Geometry check sheet. Reference: the model listing, model coordinates, mm. A direction names the side the tool comes from. Coordinates: 2 decimals unless noted, no trailing zeros. Write each loop counter-clockwise with the first axis right and the second up, starting at its lowest first coordinate (ties: lowest second). Pieces come first, ordered by that corner, then holes. Notation, with made-up numbers: (5.5, 60.25) -> (48.5, 60.25) arc R16 cw to (48.5, 64.25) -> close; hole circle Ø10 at (23.25, 41). An arc over 180 degrees is marked (long way). Answer in a Markdown table with one row per item. Add a question column.
Q1. Section check A-A, the plane z = -93. Record the boundary of the cut face in (x, y), and give its area (3 significant figures).
Q2. Tool access check on faces 1 (the face through (0, 12, -108)), 2 (the face through (-51.302, 11.832, -102.915)), 3 (the face through (72.5, 12, -38)). Record the directions out of +Z, -Z, +X, -X, +Y, -Y that give a thin tool (end or side, any length) a straight path to the whole face; none if there is none.
Q3. Section check C-C, the plane y = 13. Record the boundary of the cut face in (x, z), and give its area (3 significant figures).
Q4. Release check for a two-part mould opening along X. For faces 4 (the face through (48.698, 11.832, -102.915)), 5 (the face through (1, 0, -62)), 6 (the face through (-72.5, 12, -37)) record: pulls with the +X half, pulls with the -X half, needs draft (parallel to the pull), parting line crosses it, or undercut.
Q5. Thickness scan on line 1 (X direction, y = 16.75, z = -93); line 2 (Z direction, x = 50, y = 9.5); line 3 (X direction, y = 11, z = -99.5). Record the ranges inside material, lowest first.
Q6. Section check D-D, the plane z = -111. Record the boundary of the cut face in (x, y).
Q7. Gauge pin test, flat ends, axial feed: P1, Ø12, axis at x = 59.5, y = 6.5, coming from the -Z side; P2, Ø7, axis at y = 14, z = -23, coming from the +X side; P3, Ø10, axis at y = 17.5, z = -104, coming from the -X side; P4, Ø3, axis at x = 0.5, y = 20, coming from the +Z side. Record the tip position at first contact, or that the pin passes through.
Q8. Section check B-B, the plane x = -50. Record the boundary of the cut face in (y, z).
```python
from build123d import *

# Parameters (mm, degrees)
SKETCH1_R           = 10
BOSS_EXTRUDE1_DEPTH = 24


with BuildPart() as part:
    # Sketch1 → Boss-Extrude1 (new body)
    with BuildSketch(Plane(origin=(0, 0, 0), x_dir=(1, 0, 0), z_dir=(0, 1, 0))):
        with BuildLine():
            Line((72.5, 0), (-72.5, 0))
            Line((-72.5, 0), (-72.5, 74.703825536))
            ThreePointArc((-72.5, 74.703825536), (-66.688428669, 116.717005472), (-25.180652708, 108))
            Line((-25.180652708, 108), (25.180652708, 108))
            ThreePointArc((25.180652708, 108), (66.688428669, 116.717005472), (72.5, 74.703825536))
            Line((72.5, 74.703825536), (72.5, 0))
        make_face()
        with Locations((-50, 93)):
            Circle(SKETCH1_R, mode=Mode.SUBTRACT)
        with Locations((50, 93)):
            Circle(SKETCH1_R, mode=Mode.SUBTRACT)
    extrude(amount=BOSS_EXTRUDE1_DEPTH)


solid = part.part
```
Calculated:
| question | item | result |
|---|---|---|
| 1 | outline | (-79, 0) -> (-60, 0) -> (-60, 24) -> (-79, 24) -> close; (-40, 0) -> (40, 0) -> (40, 24) -> (-40, 24) -> close; (60, 0) -> (79, 0) -> (79, 24) -> (60, 24) -> close |
| 1 | area | 2,830 mm² |
| 2 | face 1 | -Z, +Y, -Y |
| 2 | face 2 | +Y, -Y |
| 2 | face 3 | +Z, +X, +Y, -Y |
| 3 | outline | (-72.5, -74.7) arc R29 ccw (long way) to (-25.18, -108) -> (25.18, -108) arc R29 ccw (long way) to (72.5, -74.7) -> (72.5, 0) -> (-72.5, 0) -> close; hole circle Ø20 at (-50, -93); hole circle Ø20 at (50, -93) |
| 3 | area | 16,300 mm² |
| 4 | face 4 | undercut |
| 4 | face 5 | needs draft |
| 4 | face 6 | pulls with the -X half |
| 5 | line 1 | x = -79 to -60, -40 to 40, 60 to 79 |
| 5 | line 2 | z = -122 to -103, -83 to 0 |
| 5 | line 3 | x = -78.26 to -57.6, -42.4 to 42.4, 57.6 to 78.26 |
| 6 | outline | (-72.74, 0) -> (-27.26, 0) -> (-27.26, 24) -> (-72.74, 24) -> close; (27.26, 0) -> (72.74, 0) -> (72.74, 24) -> (27.26, 24) -> close |
| 7 | P1 | stops at z = -121.79 |
| 7 | P2 | stops at x = 72.5 |
| 7 | P3 | stops at x = -78.37 |
| 7 | P4 | stops at z = 0 |
| 8 | outline | (0, -122) -> (24, -122) -> (24, -103) -> (0, -103) -> close; (0, -83) -> (24, -83) -> (24, 0) -> (0, 0) -> close |
